```python
from build123d import *

# Parameters (mm, degrees)
BOSS_EXTRUDE1_DEPTH = 2
BOSS_EXTRUDE2_DEPTH = 2
BOSS_EXTRUDE3_DEPTH = 1


with BuildPart() as part:
    # Sketch2 → Boss-Extrude1 (new body)
    with BuildSketch(Plane(origin=(0, 0, 0), x_dir=(1, 0, 0), z_dir=(0, 1, 0))):
        Polygon((-6.75, -2), (-6.75, -4), (6.75, -4), (6.75, 4), (-6.75, 4), (-6.75, 2), (-3.75, 2), (-3.75, -2), align=None)
    extrude(amount=BOSS_EXTRUDE1_DEPTH)

    # Sketch3 → Boss-Extrude2 (add)
    with BuildSketch(Plane(origin=(0, 2, 0), x_dir=(1, 0, 0), z_dir=(0, 1, 0))):
        Polygon((6.75, 4), (2.25, 4), (-0.75, 1), (-0.75, -1), (2.25, -4), (6.75, -4), align=None)
    extrude(amount=BOSS_EXTRUDE2_DEPTH)

    # Sketch5 → Boss-Extrude3 (add, symmetric)
    with BuildSketch(Plane.XY):
        Polygon((3.75, 8), (6.75, 8), (6.75, 4), (-0.75, 4), (-0.75, 5), align=None)
    extrude(amount=BOSS_EXTRUDE3_DEPTH, both=True)


solid = part.part
```
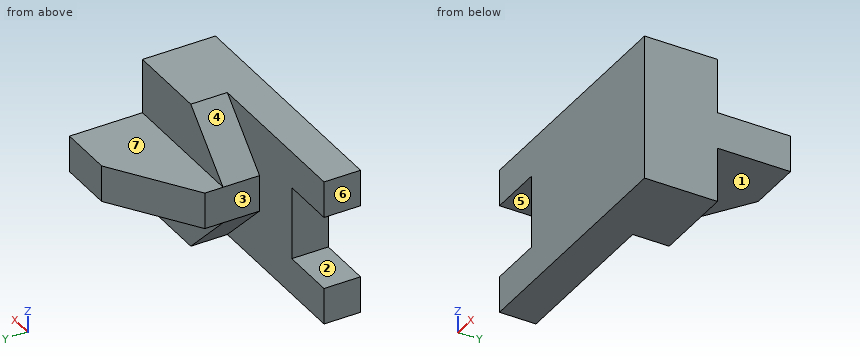
Input: part model. Units: mm. Frame: model coordinates. Face numbers are marked on the shaded views. A direction names the side the tool comes from. Give positions to 0.01 mm unless a question says otherwise; leave off trailing zeros. Write each loop counter-clockwise with the first axis right and the second up, starting at its lowest first coordinate (ties: lowest second). Pieces come first, ordered by that corner, then holes. Notation, with made-up numbers: (87.5, -26) - (94.5, -26) arc R32 cw to (94.5, 13) - close; hole circle Ø11 at (-12.75, 3). An arc over 180 degrees is marked (long way). Write item = value, one per line. Start each with the question number.
1. Section query D-D, the plane x = 5. Output: boundary loops of the cut face in (y, z).
2. Mould query, pull axis Z, two halves, no side actions, for the marked faces 5, 6 and 7. Classes: released by +Z, released by -Z, zero draft, split by the parting line, or undercut.
3. Ray query, L1, parallel to Z at x = 4.5, y = 7.25; L2, parallel to Y at x = -2, z = 3.25; L3, parallel to Y at x = 4, z = 2.5. Return the intervals inside material, ascending.
4. Section query C-C, the plane z = -1.5. Output: boundary loops of the cut face in (x, y), then the cut area to 3 significant figures.
5. Access query for the marked faces 1, 2, 3 and 4. Directions: +Z, -Z, +X, -X, +Y, -Y. A direction counts if a zero-diameter tool reaches every point of the face in a straight line with its end or side. Return the directions, or none.
6. Section query A-A, the plane x = -5.25. Output: boundary loops of the cut face in (y, z).
7. First-contact query: pin 1 Ø1.5 at (y, z) = (3, 1) entering from -X; pin 2 Ø1.5 at (x, z) = (1.5, 3) entering from +Y; pin 3 Ø0.6 at (y, z) = (1, -1) entering from -X. Flat tips, straight axial feed; report the tip coordinate or a pass-through.
8. Section query B-B, the plane y = 1. Output: boundary loops of the cut face in (x, z), then the cut area to 3 significant figures.
Check sheet entries:
q1.outline = (0, -4) - (4, -4) - (4, -1) - (8, -1) - (8, 1) - (4, 1) - (4, 4) - (0, 4) - close
q2.face_5 = undercut
q2.face_6 = zero draft
q2.face_7 = released by +Z
q3.L1 = -1 to 1
q3.L2 = 0 to 2
q3.L3 = 0 to 4
q4.outline = (-3.75, 0) - (6.75, 0) - (6.75, 4) - (-0.25, 4) - (-0.25, 2) - (-3.75, 2) - close
q4.area = 35.0 mm2
q5.face_1 = -Z, +X, -X, +Y
q5.face_2 = -X, +Y, -Y
q5.face_3 = +Z, -Z, -X, +Y
q5.face_4 = +Z, -X, +Y
q6.outline = (0, -4) - (2, -4) - (2, -2) - (0, -2) - close; (0, 2) - (2, 2) - (2, 4) - (0, 4) - close
q7.pin_1 = -0.75
q7.pin_2 = 4
q7.pin_3 = -3.75
q8.outline = (-6.75, -4) - (6.75, -4) - (6.75, 4) - (-6.75, 4) - (-6.75, 2) - (-3.75, 2) - (-3.75, -2) - (-6.75, -2) - close
q8.area = 96.0 mm2
